Can you work these out from the drawing? Everything is in mm from the part's minimum corner. A direction names the side the tool comes from. Give positions to 0.01 mm unless a question says otherwise; leave off trailing zeros. Order: outer loops, then holes, each group sorted by start corner. A loop starts at its lowest first (then second) coordinate and runs counter-clockwise, first axis right, second up. Notation, with made-up numbers: M 51.5,3 L 95.5,3 A14 cw 95.5,8 Z; hole C 69,25 d11. An arc over 180 degrees is marked long. Answer as a JSON object with one key per item and string values.
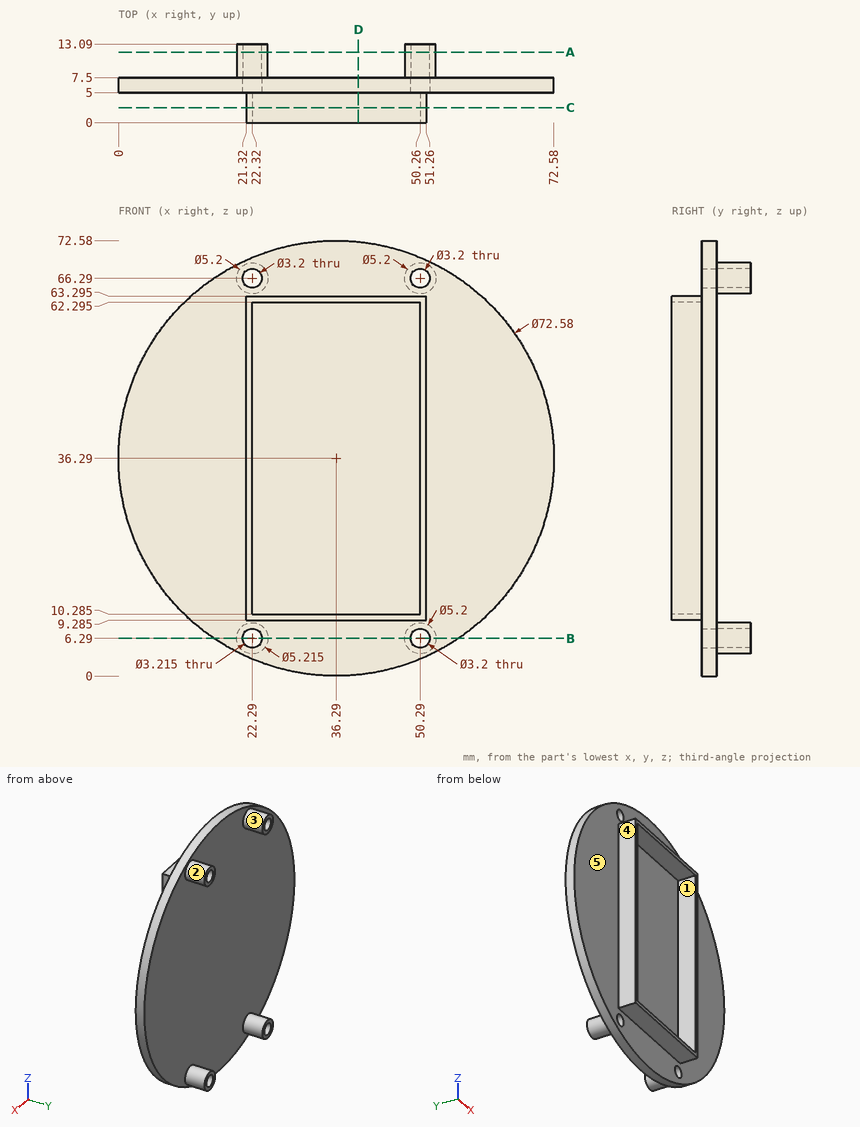
1) I want a section at D-D on x = 40. Write out the boundary of the cut face in (y, z) (1 decimal).
Results found:
{"outline": "M 0,9.3 L 5,9.3 L 5,0.2 L 7.5,0.2 L 7.5,72.4 L 5,72.4 L 5,63.3 L 0,63.3 L 0,62.3 L 5,62.3 L 5,10.3 L 0,10.3 Z"}
2) I need wall thicknesses on L1, parallel to Z at x = 50.29, y = 10; L2, parallel to X at y = 10.15, z = 6.29; L3, parallel to X at y = 2, z = 27. Which ranges of each line are inside material? Lowest first, please.
Results found:
{"L1": "z = 3.69 to 4.69, 7.89 to 8.89, 63.69 to 64.69, 67.89 to 68.89", "L2": "x = 19.68 to 20.68, 23.9 to 24.9, 47.69 to 48.69, 51.89 to 52.89", "L3": "x = 21.32 to 22.32, 50.26 to 51.26"}
3) For the marked faces 1 and 2, which set-ups out of +Z, -Z, +X, -X, +Y, -Y let a thin tool reach every point of the face, with its end or its side?
Results found:
{"face 1": "-Y", "face 2": "+Y"}
4) I want a section at C-C on y = 2.5. Write out the boundary of the cut face in (x, z) (1 decimal).
Results found:
{"outline": "M 21.3,9.3 L 51.3,9.3 L 51.3,63.3 L 21.3,63.3 Z; hole M 22.3,10.3 L 50.3,10.3 L 50.3,62.3 L 22.3,62.3 Z"}
5) Thinking about a two-plate mould opening in X: for the marked faces 3, 4 and 5, which applies, pulls with the +X half, pulls with the -X half, needs draft (parallel to the pull), parting line crosses it, or undercut?
Results found:
{"face 3": "undercut", "face 4": "pulls with the -X half", "face 5": "needs draft"}
6) I'm going to push flat-ended pins straight in: pin 1 Ø1.9 at (x, z) = (22.29, 6.29) entering from -Y; pin 2 Ø1.5 at (x, y) = (34, 1.5) entering from -Z (3 decimals); pin 3 Ø6 at (x, z) = (19.5, 19) entering from +Y; pin 4 Ø5.5 at (y, z) = (1.5, 45.5) entering from -X. Where does each tip first touch, or does it pass through?
Results found:
{"pin 1": "passes through", "pin 2": "stops at z = 9.285", "pin 3": "stops at y = 7.5", "pin 4": "stops at x = 21.32"}
7) I want a section at A-A on y = 11.75. Write out the boundary of the cut face in (x, z) (1 decimal).
Results found:
{"outline": "C 22.3,6.3 d5.2; C 22.3,66.3 d5.2; C 50.3,6.3 d5.2; C 50.3,66.3 d5.2; hole C 22.3,6.3 d3.2; hole C 22.3,66.3 d3.2; hole C 50.3,6.3 d3.2; hole C 50.3,66.3 d3.2"}
8) I want a section at B-B on z = 6.29. Write out the boundary of the cut face in (x, y).
Results found:
{"outline": "M 15.87,5 L 20.68,5 L 20.68,13.09 L 19.68,13.09 L 19.68,7.5 L 15.87,7.5 Z; M 23.9,5 L 48.69,5 L 48.69,13.09 L 47.69,13.09 L 47.69,7.5 L 24.9,7.5 L 24.9,13.09 L 23.9,13.09 Z; M 51.89,5 L 56.71,5 L 56.71,7.5 L 52.89,7.5 L 52.89,13.09 L 51.89,13.09 Z"}
